For this review, use the dimensioned drawing (mm, ordinates from the lowest corner) and the shaded views. A direction names the side the tool comes from. Give positions to 0.01 mm unless a question says otherwise; leave off trailing zeros. Loops run counter-clockwise (first coordinate to the right, second up) from the corner with the lowest first, then second, coordinate; pieces in that order, holes last. Notation, with made-up numbers: M -27.5,13.25 L 8.5,13.25 A25 ccw 8.5,39.25 Z; hole C 50,63 d5. An arc over 180 degrees is marked long. Use one line per item in the form item = value. Start each with the question number.
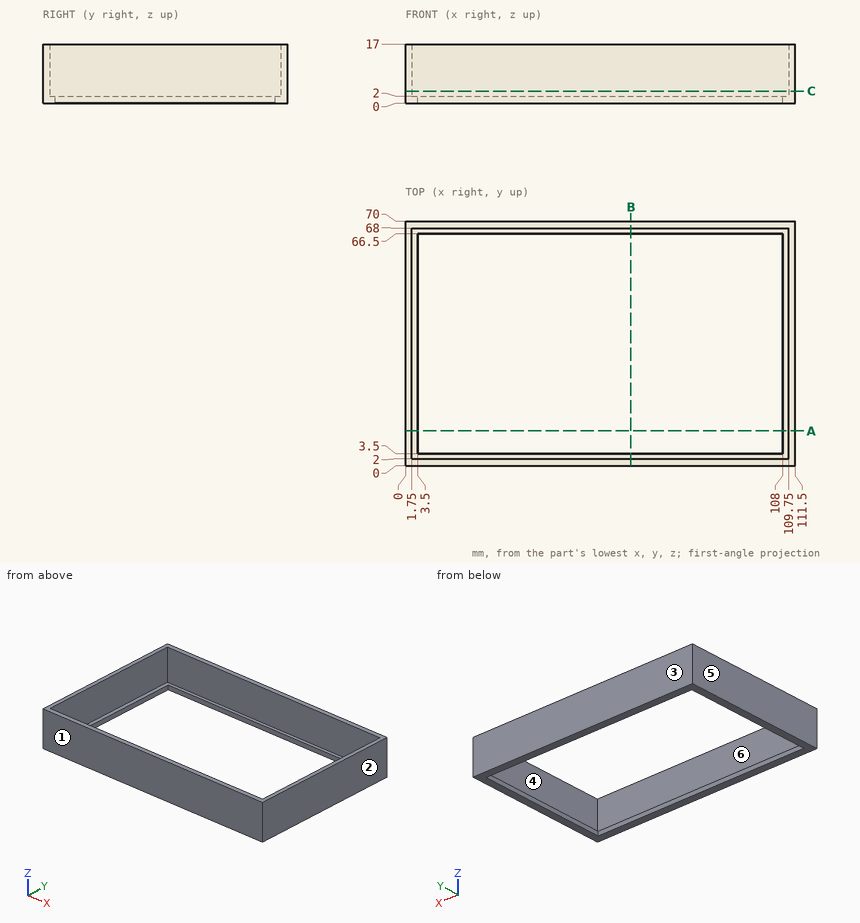
Q1. Take a section at B-B on x = 64.5. Give the boundary of the cut face in (y, z).
Q2. For the marked faces 5 and 6, list the 3-axis set-ups (+Z, -Z, +X, -X, +Y, -Y) from which the entire face can be reached by the end or side of a thin tool; tool diameter is ignored.
Q3. Take a section at C-C on z = 3.5. Give the boundary of the cut face in (x, y), plus the area to 3 significant figures.
Q4. Wall thickness on probe 1 along X at (y, z) = (63, 9.5); probe 2 along Y at (x, z) = (10, 3.75); probe 3 along Y at (x, z) = (45, 1.5): over which ranges is each line inside the solid? List them lowest first.
Q5. Take a section at A-A on y = 10. Give the boundary of the cut face in (x, z), plus the area to 3 significant figures.
Q6. The part is to be moulded in two halves that separate along Y. For the marked faces 1, 2, 3 and 4, say which applies: pulls with the +Y half, pulls with the -Y half, needs draft (parallel to the pull), parting line crosses it, or undercut.
Response values:
q1.outline = M 0,0 L 3.5,0 L 3.5,2 L 2,2 L 2,17 L 0,17 Z; M 66.5,0 L 70,0 L 70,17 L 68,17 L 68,2 L 66.5,2 Z
q2.face_5 = +Z, -Z, -X, +Y, -Y
q2.face_6 = +Z
q3.outline = M 0,0 L 111.5,0 L 111.5,70 L 0,70 Z; hole M 1.75,2 L 109.75,2 L 109.75,68 L 1.75,68 Z
q3.area = 677 mm^2
q4.probe_1 = 0 to 1.75, 109.75 to 111.5
q4.probe_2 = 0 to 2, 68 to 70
q4.probe_3 = 0 to 3.5, 66.5 to 70
q5.outline = M 0,0 L 3.5,0 L 3.5,2 L 1.75,2 L 1.75,17 L 0,17 Z; M 108,0 L 111.5,0 L 111.5,17 L 109.75,17 L 109.75,2 L 108,2 Z
q5.area = 66.5 mm^2
q6.face_1 = pulls with the -Y half
q6.face_2 = needs draft
q6.face_3 = pulls with the +Y half
q6.face_4 = undercut
